Here's how the part is built. I have some questions about the finished solid (model axes, mm). Give positions to 0.01 mm unless a question says otherwise; leave off trailing zeros. Order: outer loops, then holes, each group sorted by start corner. A loop starts at its lowest first (then second) coordinate and runs counter-clockwise, first axis right, second up.
from build123d import *

# Parameters (mm, degrees)
SKETCH_1_R      = 9.65
SKETCH_1_R_2    = 1.65
EXTRUDE_1_DEPTH = 3
FILLET_2_R      = 1
FILLET_3_R      = 0.6
FILLET_4_R      = 0.5
FILLET_5_R      = 3


with BuildPart() as part:
    # 草图1 → 凸台-拉伸1 (new body)
    with BuildSketch(Plane.XY):
        with BuildLine():
            Line((0, 0), (4, 0))
            Line((4, 0), (4, -4))
            Line((4, -4), (9.1, -4))
            Line((9.1, -4), (9.1, -9.5))
            Line((9.1, -9.5), (7.4, -9.5))
            Line((7.4, -9.5), (7.4, -12.5))
            Line((7.4, -12.5), (9.1, -12.5))
            Line((9.1, -12.5), (9.1, -17.5))
            Line((9.1, -17.5), (12.3, -17.5))
            Line((12.3, -17.5), (12.3, -12.5))
            Line((12.3, -12.5), (14, -12.5))
            Line((14, -12.5), (14, -9.5))
            Line((14, -9.5), (12.3, -9.5))
            Line((12.3, -9.5), (12.3, -4))
            Line((12.3, -4), (17.4, -4))
            Line((17.4, -4), (17.4, 0))
            Line((17.4, 0), (21.4, 0))
            Line((21.4, 0), (21.4, -4))
            Line((21.4, -4), (21.4, -19))
            Line((21.4, -19), (16.4, -19))
            Line((16.4, -19), (16.4, -40.956914646))
            ThreePointArc((16.4, -40.956914646), (22.95, -51.8), (16.4, -62.643085354))
            Line((16.4, -62.643085354), (16.4, -81.843085354))
            Line((16.4, -81.843085354), (5, -81.843085354))
            Line((5, -81.843085354), (5, -62.643085354))
            ThreePointArc((5, -62.643085354), (-1.55, -51.8), (5, -40.956914646))
            Line((5, -40.956914646), (5, -19))
            Line((5, -19), (0, -19))
            Line((0, -19), (0, -4))
            Line((0, -4), (0, 0))
        make_face()
        with Locations((10.7, -51.8)):
            Circle(SKETCH_1_R, mode=Mode.SUBTRACT)
        with Locations((10.7, -25.8)):
            Circle(SKETCH_1_R_2, mode=Mode.SUBTRACT)
        with Locations((10.7, -77.8)):
            Circle(SKETCH_1_R_2, mode=Mode.SUBTRACT)
    extrude(amount=EXTRUDE_1_DEPTH)

    # 圆角2
    fillet_2_edges = [part.edges().sort_by_distance(p)[0] for p in [
        (21.4, -19, 1.5),
        (16.4, -19, 1.5),
        (5, -19, 1.5),
        (0, -19, 1.5),
    ]]
    fillet(fillet_2_edges, radius=FILLET_2_R)

    # 圆角3
    fillet_3_edges = [part.edges().sort_by_distance(p)[0] for p in [
        (9.1, -4, 1.5),
        (12.3, -4, 1.5),
    ]]
    fillet(fillet_3_edges, radius=FILLET_3_R)

    # 圆角4
    fillet_4_edges = [part.edges().sort_by_distance(p)[0] for p in [
        (0, 0, 1.5),
        (4, 0, 1.5),
        (17.4, 0, 1.5),
        (21.4, 0, 1.5),
    ]]
    fillet(fillet_4_edges, radius=FILLET_4_R)

    # 圆角5
    fillet_5_edges = [part.edges().sort_by_distance(p)[0] for p in [
        (16.4, -40.956914646, 1.5),
        (16.4, -62.643085354, 1.5),
        (5, -62.643085354, 1.5),
        (5, -40.956914646, 1.5),
    ]]
    fillet(fillet_5_edges, radius=FILLET_5_R)


solid = part.part
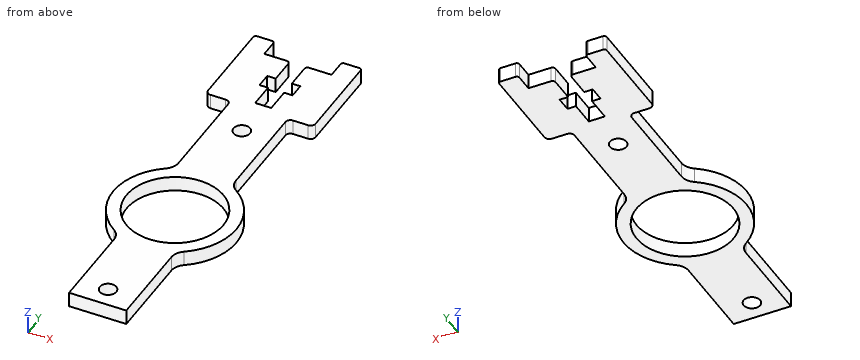
Q1. If we section it at C-C on x = 6.25: List the corners of the cut face in (y, z) for me, plus the area to 3 significant figures.
Filled sheet:
outline: (-81.84, 0) - (-60.36, 0) - (-60.36, 3) - (-81.84, 3) - close; (-43.24, 0) - (-4, 0) - (-4, 3) - (-43.24, 3) - close
area: 182 mm2
Q2. I'm going to push flat-ended pins straight in: P1, Ø1.5, axis at x = 19.5, z = 1.5, coming from the -Y side; P2, Ø0.8, axis at x = 13.5, z = 1, coming from the +Y side; P3, Ø1.5, axis at x = 3.5, y = -24.5, coming from the -Z side; P4, Ø0.9, axis at y = -11.5, z = 1, coming from the -X side. Where does each tip first touch, or does it pass through?
Filled sheet:
P1: stops at y = -61.03
P2: stops at y = -4
P3: passes through
P4: stops at x = 0
Q3. I need wall thicknesses on L1, parallel to Y at x = 10.7, z = 1.1; L2, parallel to Y at x = 4.25, z = 1.4; L3, parallel to Y at x = 18.5, z = 1.05. Which ranges of each line are inside material? Lowest first, please.
Filled sheet:
L1: y = -81.84 to -79.45, -76.15 to -61.45, -42.15 to -27.45, -24.15 to -17.5
L2: y = -62.34 to -58.98, -44.62 to -41.26, -19.03 to -4
L3: y = -61.25 to -57.48, -46.12 to -42.35, -19 to 0
Q4. If we section it at D-D on z = 1.05: Give the number of separate pieces and of enclosed holes in the cut face, plus the area to 3 significant figures.
Filled sheet:
separate pieces: 1
enclosed holes: 3
area: 910 mm2
Q5. If we section it at B-B on x = 10.7: List the corners of the cut face in (y, z) for me.
Filled sheet:
outline: (-81.84, 0) - (-79.45, 0) - (-79.45, 3) - (-81.84, 3) - close; (-76.15, 0) - (-61.45, 0) - (-61.45, 3) - (-76.15, 3) - close; (-42.15, 0) - (-27.45, 0) - (-27.45, 3) - (-42.15, 3) - close; (-24.15, 0) - (-17.5, 0) - (-17.5, 3) - (-24.15, 3) - close
Q6. If we section it at A-A on y = -25.8: List the corners of the cut face in (x, z) for me, plus the area to 3 significant figures.
Filled sheet:
outline: (5, 0) - (9.05, 0) - (9.05, 3) - (5, 3) - close; (12.35, 0) - (16.4, 0) - (16.4, 3) - (12.35, 3) - close
area: 24.3 mm2
